Read the model definition and answer for the solid it produces. Units are mm, in the model's axes. Face numbers are marked on the shaded views. A direction names the side the tool comes from. Coordinates: 2 decimals unless noted, no trailing zeros. Loops run counter-clockwise (first coordinate to the right, second up) from the corner with the lowest first, then second, coordinate; pieces in that order, holes last. Notation, with made-up numbers: (89.5, 33) -> (109.5, 33) arc R16 ccw to (109.5, 59) -> close; hole circle Ø8 at (22, 56.5). An arc over 180 degrees is marked (long way). Answer in a Markdown table with one row per item.
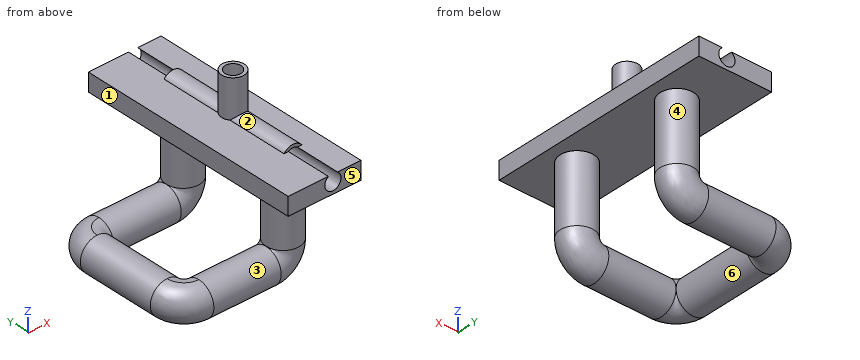
Autodesk Inventor part; units mm, degrees
ref_plane "YZ Plane" through (0, 0, 0) normal (1, 0, 0) x (0, 1, 0)
ref_plane "XZ Plane" through (0, 0, 0) normal (0, 1, 0) x (-1, 0, 0)
sketch "Sketch1" plane through (0, 0, 0) normal (0, 1, 0) x (-1, 0, 0)
  circle A0 centre (0, 0) radius 3.575
  circle A1 centre (0, 0) radius 5
  dimension "d0" = 7.15
  dimension "d1" = 10
extrude "Extrusion1" add sketch "Sketch1" along normal mid plane 60
ref_plane "Work Plane1" through (0, 0, 5) normal (0, 0, 1) x (1, 0, 0)
sketch "Sketch2" plane through (0, 0, 5) normal (0, 0, 1) x (1, 0, 0)
  circle A0 centre (0, 0) radius 3.575
  circle A1 centre (0, 0) radius 5
  line L0 (5, 30) -> (-5, 30)
  dimension "d4" = 7.15
  dimension "d5" = 10
  dimension "d22" = 0
extrude "Extrusion2" add sketch "Sketch2" along normal blind 15 and the other way blind 5
sketch "Sketch3" plane through (0, 0, 20) normal (0, 0, 1) x (1, 0, 0)
  circle A0 centre (0, 0) radius 3.575
extrude "Extrusion3" cut sketch "Sketch3" against normal up to surface
sketch "Sketch4" plane through (0, 30, 0) normal (0, 1, 0) x (1, 0, 0)
  circle A0 centre (0, 0) radius 3.675
  dimension "d13" = 7.35
extrude "Extrusion4" cut sketch "Sketch4" against normal through all
ref_plane "Work Plane3" through (0, 0, -5) normal (0, 0, 1) x (1, 0, 0)
sketch "Sketch6" plane through (0, 0, -5) normal (0, 0, 1) x (1, 0, 0)
  line L0 (12.5, -50) -> (-12.5, -50)
  line L1 (-12.5, -50) -> (-12.5, 50)
  line L2 (-12.5, 50) -> (12.5, 50)
  line L3 (12.5, 50) -> (12.5, -50)
  line L4 (12.5, -50) -> (-12.5, 50) construction
  line L5 (-12.5, -50) -> (12.5, 50) construction
  point P0 (0, 0)
  dimension "d23" = 25
  dimension "d24" = 100
extrude "Extrusion6" add sketch "Sketch6" along normal blind 8
sketch "Sketch7" plane through (0, -30, 0) normal (0, -1, 0) x (1, 0, 0)
  circle A0 centre (0, 0) radius 3.615
  dimension "d27" = 7.23
extrude "Extrusion7" cut sketch "Sketch7" along normal through all both and the other way through all
sketch "Sketch8" plane through (0, 0, -5) normal (0, 0, -1) x (-1, 0, 0)
  circle A0 centre (0, -25) radius 7.5
  circle A1 centre (0, 25) radius 7.5
  point P0 (0, 0)
  dimension "d30" = 15
  dimension "d31" = 15
  dimension "d32" = 50
  dimension "d33" = 25
extrude "Extrusion8" add sketch "Sketch8" along normal blind 30
sketch "Sketch9" plane through (0, 25, -35) normal (0, 0, -1) x (-1, 0, 0)
  circle A0 centre (0, 0) radius 7.5
  line L0 (7.5, 0) -> (7.5, -9.7245)
  line L1 (7.5, -9.7245) -> (7.5, 12.7829)
  point P0 (0, -25)
revolve "Revolution1" add sketch "Sketch9" angle 90 about axis through (-7.5, 15.2755, -35) along (0, 1, 0)
mirror "Mirror1" about plane through (0, 0, 0) normal (0, 1, 0) of "Revolution1"
sketch "Sketch10" plane through (-7.5, 25, -42.5) normal (-1, 0, 0) x (0, 0, 1)
  circle A0 centre (0, 0) radius 7.5
  point P0 (42.5, -25)
  dimension "d37" = 15
extrude "Extrusion9" add sketch "Sketch10" along normal blind 30
mirror "Mirror2" about plane through (0, 0, 0) normal (0, 1, 0) of "Extrusion9"
sketch "Sketch11" plane through (-37.5, 25, -42.5) normal (-1, 0, 0) x (0, 0, 1)
  circle A0 centre (0, 0) radius 7.5
  circle A1 centre (0, 0) radius 7.5
  line L0 (0, -7.5) -> (-9.6615, -7.5)
  line L1 (-9.6615, -7.5) -> (9.5932, -7.5)
  point P0 (42.5, -25)
  dimension "d40" = 15
sketch "Sketch12" plane through (-37.5, -25, -42.5) normal (-1, 0, 0) x (0, 0, 1)
  circle A0 centre (0, 0) radius 7.5
  line L0 (0, 7.5) -> (-6.8839, 7.5)
  circle A1 centre (0, 0) radius 7.5
  line L1 (-6.8839, 7.5) -> (7.5, 7.5)
  point P0 (42.5, 25)
  dimension "d41" = 15
revolve "Revolution2" add sketch "Sketch12" angle 90 about axis through (-37.5, -17.5, -49.3839) along (0, 0, -1)
mirror "Mirror3" about plane through (0, 0, 0) normal (0, 1, 0) of "Revolution2"
sketch "Sketch13" plane through (-45, 17.5, -42.5) normal (0, -1, 0) x (1, 0, 0)
  circle A0 centre (0, 0) radius 7.5
  point P0 (45, 42.5)
  dimension "d43" = 15
extrude "Extrusion10" add sketch "Sketch13" along normal up to surface (35 mm away)
sketch "Sketch14" plane through (-12.5, -50, -5) normal (-1, 0, 0) x (0, 0, 1)
  line L0 (0, 100) -> (0, 0)
  line L1 (8, 100) -> (8, 0)
  line L2 (0, 0) -> (8, 0)
  line L3 (8, 0) -> (8, 100)
  line L4 (8, 100) -> (0, 100)
  line L5 (0, 100) -> (0, 0)
  point P0 (5, 50)
extrude "Extrusion11" add sketch "Sketch14" along normal blind 7.5
sketch "Sketch5" plane through (0, 0, -5) normal (0, 0, 1) x (1, 0, 0)
  line L0 (5, 15) -> (-5, 15)
  line L1 (-5, -15) -> (5, -15)
  line L2 (2, 15) -> (-2, 15)
  line L3 (-2, 15) -> (-2, -15)
  line L4 (-2, -15) -> (2, -15)
  line L5 (2, -15) -> (2, 15)
  point P0 (0, 0)
  dimension "d16" = 4
  dimension "d17" = 2
properties part number "T-joint_hand"
1. The mould has two halves that part along Z. Classify the marked faces 4, 5 and 6: pulls with the +Z half, pulls with the -Z half, needs draft (parallel to the pull), parting line crosses it, or undercut.
A:
| item | result |
|---|---|
| face 4 | undercut |
| face 5 | needs draft |
| face 6 | parting line crosses it |
2. A cutting plane is placed at A-A on y = -16. Give the vertices of the cut face in (x, z) (3 decimals).
A:
| item | result |
|---|---|
| outline | circle Ø15 at (-45, -42.5); (-20, -5) -> (12.5, -5) -> (12.5, 3) -> (4, 3) arc R5 ccw to (-4, 3) -> (-20, 3) -> close; hole (-2.123, 3) -> (-2.017, 3) arc R3.615 ccw (long way) to (2.017, 3) -> (2.123, 3) arc R3.675 ccw to start |
3. A cutting plane is placed at C-C on x = -11. Give the vertices of the cut face in (y, z).
A:
| item | result |
|---|---|
| outline | (-50, -5) -> (50, -5) -> (50, 3) -> (-50, 3) -> close; circle Ø15 at (-25, -42.5); circle Ø15 at (25, -42.5) |
4. A tool of negligible diameter and unlimited length cuts with its end or side. For the marked faces 1, 2 and 3, from which of +Z, -Z, +X, -X, +Y, -Y can it reach the whole face along a straight path? Write none if from no direction.
A:
| item | result |
|---|---|
| face 1 | +Z, -X, +Y, -Y |
| face 2 | +Z, -Y |
| face 3 | none |
5. Given pin 1 Ø3 at (x, y) = (-40, 27) entering from -Z; pin 2 Ø14.5 at (x, y) = (-15, -17.5) entering from +Z; pin 3 Ø0.6 at (x, z) = (1, 4) entering from +Y, each flat-ended and moving along its own axis, determine where each tip first touches the part or whether it passes through.
A:
| item | result |
|---|---|
| pin 1 | stops at z = -49.95 |
| pin 2 | stops at z = 3 |
| pin 3 | stops at y = 30 |
6. Find the intervals of material crossed by probe 1 along Y at (x, z) = (0, 11.5) (3 decimals); probe 2 along X at (y, z) = (27, 0) (3 decimals), in increasing order.
A:
| item | result |
|---|---|
| probe 1 | y = -5 to -3.575, 3.575 to 5 |
| probe 2 | x = -20 to -3.615, 3.615 to 12.5 |
7. A cutting plane is placed at D-D on y = 0. Give the vertices of the cut face in (x, z) (3 decimals), and give its area (3 significant figures).
A:
| item | result |
|---|---|
| outline | circle Ø15 at (-45, -42.5); (-20, -5) -> (12.5, -5) -> (12.5, 3) -> (5, 3) -> (5, 20) -> (3.575, 20) -> (3.575, 3) -> (2.017, 3) arc R3.615 cw (long way) to (-2.017, 3) -> (-3.575, 3) -> (-3.575, 20) -> (-5, 20) -> (-5, 3) -> (-20, 3) -> close |
| area | 446 mm2 |
8. A cutting plane is placed at B-B on z = 0. Give the vertices of the cut face in (x, y) (3 decimals), and give its area (3 significant figures).
A:
| item | result |
|---|---|
| outline | (-20, -50) -> (-3.615, -50) -> (-3.615, 50) -> (-20, 50) -> close; (3.615, -50) -> (12.5, -50) -> (12.5, 50) -> (3.615, 50) -> close |
| area | 2,530 mm2 |
